Answer from the drawing. Dimensions are ordinates in mm from the lowest x, y and z of the part. A direction names the side the tool comes from. Round coordinates to 2 decimals unless told otherwise and drop trailing zeros. Write each loop counter-clockwise with the first axis right and the second up, starting at its lowest first coordinate (ties: lowest second). Pieces come first, ordered by that corner, then holes. Notation, with made-up numbers: (21.5, 83) - (45.5, 83) arc R16 ccw to (45.5, 114) - close; hole circle Ø4 at (35, 84). An arc over 180 degrees is marked (long way). Use a Markdown table: item, result. Add a question column.
1) Each of these flat-tipped pins is pushed along its axis until it touches: P1, Ø3.5, axis at x = 20, y = 5, coming from the +Z side; P2, Ø3.5, axis at x = 5, y = 5, coming from the +Z side; P3, Ø1.5, axis at x = 22, z = 7, coming from the -Y side. Where does it stop, or does it pass through?
2) Determine the mould class of the marked faces 1, 2 and 3 for opening direction Y: +Y half, -Y half, draft (parallel to the pull), parting line (faces both ways), or undercut.
3) A cutting plane is placed at A-A (y = 5). Give the vertices of the cut face in (x, z), then the cut area to 3 significant figures.
4) A cutting plane is placed at B-B (x = 5). Give the vertices of the cut face in (y, z), then the cut area to 3 significant figures.
5) A cutting plane is placed at D-D (z = 8.75). Give the vertices of the cut face in (x, y), then the cut area to 3 significant figures.
6) A cutting plane is placed at C-C (z = 3.25). Give the vertices of the cut face in (x, y), then the cut area to 3 significant figures.
7) Find the intervals of material crossed by probe 1 along X at (y, z) = (5, 2.8); probe 2 along Y at (x, z) = (20, 2.6); probe 3 along Y at (x, z) = (5, 2.7), in increasing order. Write a range as from..to.
8) A tool of negligible diameter and unlimited length cuts with its end or side. For the marked faces 4 and 5, from which of +Z, -Z, +X, -X, +Y, -Y can it reach the whole face along a straight path? Write none if from no direction.
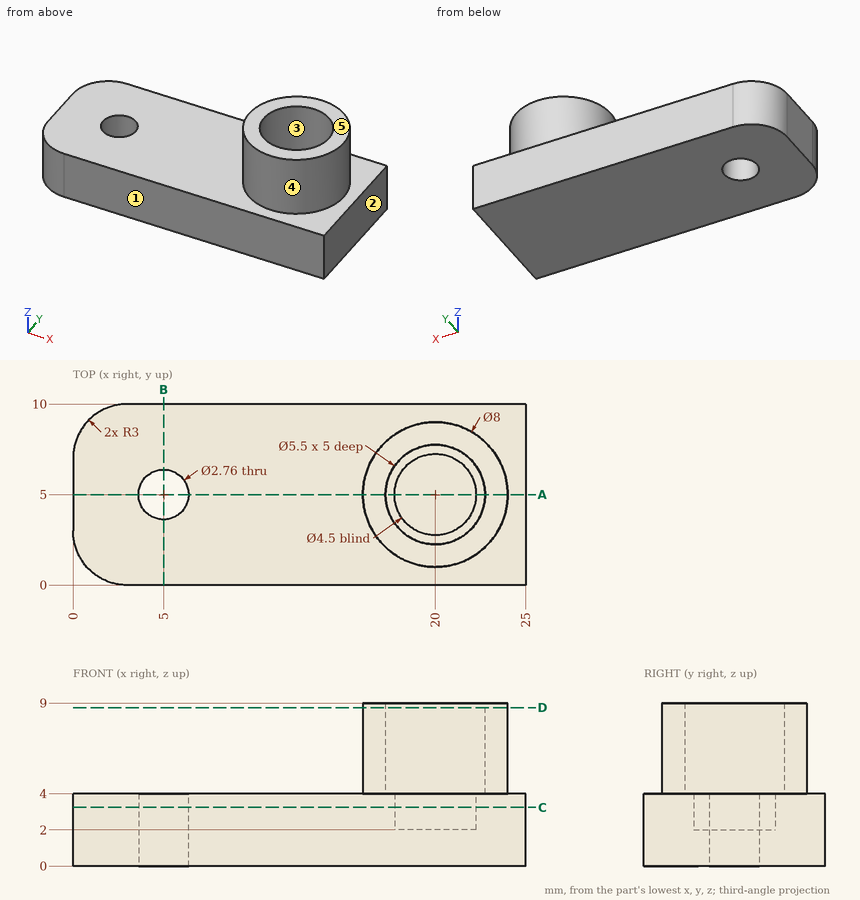
Entries:
| question | item | result |
|---|---|---|
| 1 | P1 | stops at z = 2 |
| 1 | P2 | stops at z = 4 |
| 1 | P3 | stops at y = 1.2 |
| 2 | face 1 | -Y half |
| 2 | face 2 | draft |
| 2 | face 3 | undercut |
| 3 | outline | (0, 0) - (3.62, 0) - (3.62, 4) - (0, 4) - close; (6.38, 0) - (25, 0) - (25, 4) - (24, 4) - (24, 9) - (22.75, 9) - (22.75, 4) - (22.25, 4) - (22.25, 2) - (17.75, 2) - (17.75, 4) - (17.25, 4) - (17.25, 9) - (16, 9) - (16, 4) - (6.38, 4) - close |
| 3 | area | 92.5 mm² |
| 4 | outline | (0, 0) - (3.62, 0) - (3.62, 4) - (0, 4) - close; (6.38, 0) - (10, 0) - (10, 4) - (6.38, 4) - close |
| 4 | area | 29.0 mm² |
| 5 | outline | circle Ø8 at (20, 5); hole circle Ø5.5 at (20, 5) |
| 5 | area | 26.5 mm² |
| 6 | outline | (0, 3) arc R3 ccw to (3, 0) - (25, 0) - (25, 10) - (3, 10) arc R3 ccw to (0, 7) - close; hole circle Ø2.76 at (5, 5); hole circle Ø4.5 at (20, 5) |
| 6 | area | 224 mm² |
| 7 | probe 1 | x = 0..3.62, 6.38..17.75, 22.25..25 |
| 7 | probe 2 | y = 0..2.75, 7.25..10 |
| 7 | probe 3 | y = 0..3.62, 6.38..10 |
| 8 | face 4 | +Z |
| 8 | face 5 | +Z, +X, -X, +Y, -Y |
